Verification items for the finished model (mm, model axes). Face numbers are marked on the shaded views. A direction names the side the tool comes from. Give positions to 0.01 mm unless a question says otherwise; leave off trailing zeros. Write each loop counter-clockwise with the first axis right and the second up, starting at its lowest first coordinate (ties: lowest second). Pieces come first, ordered by that corner, then holes. Notation, with made-up numbers: (-32, 58) - (22, 58) arc R9 ccw to (22, 62) - close; hole circle Ø4 at (-4, 70). An arc over 180 degrees is marked (long way). Answer as a JSON object with one key per item and string values. Group by question number.
Item 1: Sectioned sample at D-D, the plane y = 26. Record the boundary of the cut face in (x, z), and give its area (3 significant figures).
Item 2: Draft check along X on the marked faces 1, 2, 3 and 4. Enter one of: +X half, -X half, draft (parallel to the pull), parting line (faces both ways), or undercut.
Item 3: Scan lines: line 1 along Z through (x, y) = (81.5, -1.5); line 2 along X through (y, z) = (13.5, -5.5); line 3 along Y through (x, z) = (38.5, -37.5). Record each from-to range of solid material in increasing order. Write a range as [from, to].
Item 4: Tool access check on the marked faces 5, 6 and 7. Record the directions out of +Z, -Z, +X, -X, +Y, -Y that give a thin tool (end or side, any length) a straight path to the whole face; none if there is none.
Item 5: Sectioned sample at A-A, the plane y = 56.5. Record the boundary of the cut face in (x, z), and give its area (3 significant figures).
Item 6: Sectioned sample at B-B, the plane x = 50. Record the boundary of the cut face in (y, z).
Item 7: Sectioned sample at C-C, the plane z = -7. Record the boundary of the cut face in (x, y).
Item 8: Go/stop test with flat-tipped pins: pin 1 (8 mm diameter, centred on x = -108, z = -33, fed in from +Y); pin 2 (3 mm diameter, centred on x = -90.5, y = 8, fed in from -Z); pin 3 (10 mm diameter, centred on x = -123.5, y = -10.5, fed in from -Z); pin 4 (6 mm diameter, centred on x = 107.73, z = 16.4, fed in from -Y). Record where each tip stops, or that it passes through.
```python
from build123d import *

# Parameters (mm, degrees)
BOSS_EXTRUDE1_DEPTH = 10
CUT_EXTRUDE1_DEPTH  = 9.5
SKETCH3_R           = 0.15
SKETCH3_R_2         = 0.5
CUT_EXTRUDE2_DEPTH  = 20.798989873
SKETCH4_R           = 0.1
SKETCH4_W           = 8.7
SKETCH4_H           = 5.3
CUT_EXTRUDE3_DEPTH  = 20.798989873
CUT_EXTRUDE5_REACH  = 24.361
SKETCH5_W           = 20
SKETCH5_H           = 9
BOSS_EXTRUDE5_START = 9.5
SKETCH6_W           = 3.5
SKETCH6_H           = 1
BOSS_EXTRUDE5_DEPTH = 9.5
SCALE2_SCALE        = 10
SKETCH9_R           = 1.5
CUT_EXTRUDE6_DEPTH  = 10


with BuildPart() as part:
    # Sketch1 → Boss-Extrude1 (new body)
    with BuildSketch(Plane(origin=(0, 0, 0), x_dir=(1, 0, 0), z_dir=(0, 1, 0))):
        with BuildLine():
            Line((-10, 6), (10, 6))
            ThreePointArc((10, 6), (16, 0), (10, -6))
            Line((10, -6), (-10, -6))
            ThreePointArc((-10, -6), (-16, 0), (-10, 6))
        make_face()
    extrude(amount=BOSS_EXTRUDE1_DEPTH)

    # Sketch2 → Cut-Extrude1 (cut)
    with BuildSketch(Plane(origin=(0, 10, 0), x_dir=(1, 0, 0), z_dir=(0, 1, 0))):
        with BuildLine():
            Line((-10, 5.5), (10, 5.5))
            ThreePointArc((10, 5.5), (15.5, 0), (10, -5.5))
            Line((10, -5.5), (-10, -5.5))
            ThreePointArc((-10, -5.5), (-15.5, 0), (-10, 5.5))
        make_face()
    extrude(amount=-CUT_EXTRUDE1_DEPTH, mode=Mode.SUBTRACT)

    # Sketch3 → Cut-Extrude2 (cut, through all)
    with BuildSketch(Plane.XZ):
        with Locations(Location((-13, 3, 0), (0, 0, 270))):
            Circle(SKETCH3_R)
        with Locations(Location((-7, 3, 0), (0, 0, 270))):
            Circle(SKETCH3_R)
        with Locations(Location((-13, -3, 0), (0, 0, 270))):
            Circle(SKETCH3_R)
        with Locations(Location((-7, -3, 0), (0, 0, 270))):
            Circle(SKETCH3_R)
        with Locations(Location((-12.5, 0, 0), (0, 0, 270))):
            Circle(SKETCH3_R_2)
        with Locations(Location((-12.022542486, 1.469463131, 0), (0, 0, 270))):
            Circle(SKETCH3_R_2)
        with Locations(Location((-10.772542486, 2.377641291, 0), (0, 0, 270))):
            Circle(SKETCH3_R_2)
        with Locations(Location((-9.227457514, 2.377641291, 0), (0, 0, 270))):
            Circle(SKETCH3_R_2)
        with Locations(Location((-7.977457514, 1.469463131, 0), (0, 0, 270))):
            Circle(SKETCH3_R_2)
        with Locations(Location((-7.5, 0, 0), (0, 0, 270))):
            Circle(SKETCH3_R_2)
        with Locations(Location((-7.977457514, -1.469463131, 0), (0, 0, 270))):
            Circle(SKETCH3_R_2)
        with Locations(Location((-9.227457514, -2.377641291, 0), (0, 0, 270))):
            Circle(SKETCH3_R_2)
        with Locations(Location((-10.772542486, -2.377641291, 0), (0, 0, 270))):
            Circle(SKETCH3_R_2)
        with Locations(Location((-12.022542486, -1.469463131, 0), (0, 0, 270))):
            Circle(SKETCH3_R_2)
        with Locations(Location((12.022542486, -1.469463131, 0), (0, 0, 90))):
            Circle(SKETCH3_R_2)
        with Locations(Location((10.772542486, -2.377641291, 0), (0, 0, 90))):
            Circle(SKETCH3_R_2)
        with Locations(Location((9.227457514, -2.377641291, 0), (0, 0, 90))):
            Circle(SKETCH3_R_2)
        with Locations(Location((7.977457514, -1.469463131, 0), (0, 0, 90))):
            Circle(SKETCH3_R_2)
        with Locations(Location((7.5, 0, 0), (0, 0, 90))):
            Circle(SKETCH3_R_2)
        with Locations(Location((7.977457514, 1.469463131, 0), (0, 0, 90))):
            Circle(SKETCH3_R_2)
        with Locations(Location((9.227457514, 2.377641291, 0), (0, 0, 90))):
            Circle(SKETCH3_R_2)
        with Locations(Location((10.772542486, 2.377641291, 0), (0, 0, 90))):
            Circle(SKETCH3_R_2)
        with Locations(Location((12.022542486, 1.469463131, 0), (0, 0, 90))):
            Circle(SKETCH3_R_2)
        with Locations(Location((12.5, 0, 0), (0, 0, 90))):
            Circle(SKETCH3_R_2)
        with Locations(Location((7, -3, 0), (0, 0, 90))):
            Circle(SKETCH3_R)
        with Locations(Location((13, -3, 0), (0, 0, 90))):
            Circle(SKETCH3_R)
        with Locations(Location((7, 3, 0), (0, 0, 90))):
            Circle(SKETCH3_R)
        with Locations(Location((13, 3, 0), (0, 0, 90))):
            Circle(SKETCH3_R)
    extrude(amount=-CUT_EXTRUDE2_DEPTH, mode=Mode.SUBTRACT)

    # Sketch4 → Cut-Extrude3 (cut, through all)
    with BuildSketch(Plane.XZ):
        with Locations(Location((-4.572, 2.794, 0), (0, 0, 270))):
            Circle(SKETCH4_R)
        with Locations(Location((4.572, 2.794, 0), (0, 0, 270))):
            Circle(SKETCH4_R)
        with Locations(Location((-4.572, -2.794, 0), (0, 0, 270))):
            Circle(SKETCH4_R)
        with Locations(Location((4.572, -2.794, 0), (0, 0, 270))):
            Circle(SKETCH4_R)
        Rectangle(SKETCH4_W, SKETCH4_H)
    extrude(amount=-CUT_EXTRUDE3_DEPTH, mode=Mode.SUBTRACT)

    # Cut-Extrude5: up to this face of the body (flat: up to its plane)
    cut_extrude5_end = Plane(part.part.faces().sort_by_distance((0, 5.25, -5.5))[0])
    # Sketch5 → Cut-Extrude5 (cut, up to the picked face)
    with BuildSketch(Plane(origin=(0, 0, -6), x_dir=(-1, 0, 0), z_dir=(0, 0, -1)), mode=Mode.PRIVATE) as cut_extrude5_sk1:
        with Locations((0, 5.5)):
            Rectangle(SKETCH5_W, SKETCH5_H)
    cut_extrude5_tool1 = split(extrude(cut_extrude5_sk1.sketch, amount=-CUT_EXTRUDE5_REACH, mode=Mode.PRIVATE), bisect_by=cut_extrude5_end, keep=Keep.BOTH, mode=Mode.PRIVATE)
    add(cut_extrude5_tool1.solids().sort_by(Axis((0, 5.5, -6), (0, 0, 1)))[0], mode=Mode.SUBTRACT)

    # Sketch6 → Boss-Extrude5 (add)
    with BuildSketch(Plane(origin=(0, 0.5, 0), x_dir=(1, 0, 0), z_dir=(0, 1, 0)).offset(BOSS_EXTRUDE5_START)):
        with Locations((8.25, -5)):
            Rectangle(SKETCH6_W, SKETCH6_H)
        with Locations((8.25, 5)):
            Rectangle(SKETCH6_W, SKETCH6_H)
        with BuildLine():
            ThreePointArc((13.16227766, 4.5), (11.658312395, 5.244044241), (10, 5.5))
            Line((10, 5.5), (10, 4.5))
            Line((10, 4.5), (13.16227766, 4.5))
        make_face()
        with BuildLine():
            ThreePointArc((10, -5.5), (11.658312395, -5.244044241), (13.16227766, -4.5))
            Line((13.16227766, -4.5), (10, -4.5))
            Line((10, -4.5), (10, -5.5))
        make_face()
        with Locations((-8.25, -5)):
            Rectangle(SKETCH6_W, SKETCH6_H)
        with Locations((-8.25, 5)):
            Rectangle(SKETCH6_W, SKETCH6_H)
        with BuildLine():
            Line((-10, 4.5), (-10, 5.5))
            ThreePointArc((-10, 5.5), (-11.658312395, 5.244044241), (-13.16227766, 4.5))
            Line((-13.16227766, 4.5), (-10, 4.5))
        make_face()
        with BuildLine():
            Line((-10, -4.5), (-13.16227766, -4.5))
            ThreePointArc((-13.16227766, -4.5), (-11.658312395, -5.244044241), (-10, -5.5))
            Line((-10, -5.5), (-10, -4.5))
        make_face()
    extrude(amount=-BOSS_EXTRUDE5_DEPTH)


with BuildPart() as part_1:
    # Scale2: scaled about (0, 4.064159542, 0.819354557)
    add(part.part.scale(SCALE2_SCALE).moved(Location((0, -36.577435878, -7.374191013))))

    # Sketch9 → Cut-Extrude6 (cut)
    with BuildSketch(Plane(origin=(0, 63.422564119, 0), x_dir=(1, 0, 0), z_dir=(0, 1, 0))):
        with Locations(Location((-110, 57.374191011, 0), (0, 0, 270))):
            Circle(SKETCH9_R)
        with Locations(Location((-110, -42.625808989, 0), (0, 0, 270))):
            Circle(SKETCH9_R)
        with Locations(Location((110, -42.625808989, 0), (0, 0, 270))):
            Circle(SKETCH9_R)
        with Locations(Location((110, 57.374191011, 0), (0, 0, 270))):
            Circle(SKETCH9_R)
    extrude(amount=-CUT_EXTRUDE6_DEPTH, mode=Mode.SUBTRACT)


solid = part_1.part
```
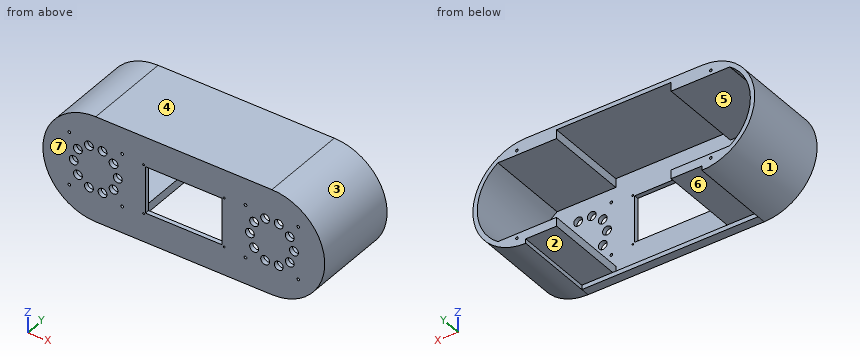
Geometry check:
{
 "1": {"outline": "(-131.62, -52.37) arc R55 cw to (-131.62, 37.63) - (-65, 37.63) - (-65, 47.63) - (65, 47.63) - (65, 37.63) - (131.62, 37.63) arc R55 cw to (131.62, -52.37) - (65, -52.37) - (65, -62.37) - (100, -62.37) - (100, -67.37) arc R60 ccw to (100, 52.63) - (-100, 52.63) arc R60 ccw to (-100, -67.37) - (-100, -62.37) - (-65, -62.37) - (-65, -52.37) - close", "area": "5,070 mm^2"},
 "2": {"face 1": "-X half", "face 2": "undercut", "face 3": "+X half", "face 4": "draft"},
 "3": {"line 1": "[-62.37, -52.37], [37.63, 52.63]", "line 2": "[-159.97, -154.97], [154.97, 159.97]", "line 3": "[-36.58, -31.58]"},
 "4": {"face 5": "+Y", "face 6": "-Z, +Y", "face 7": "+Z, -Z, +X, -X, -Y"},
 "5": {"outline": "(-131.62, -52.37) arc R55 cw to (-131.62, 37.63) - (-65, 37.63) - (-65, 47.63) - (65, 47.63) - (65, 37.63) - (131.62, 37.63) arc R55 cw to (131.62, -52.37) - (65, -52.37) - (65, -62.37) - (100, -62.37) - (100, -67.37) arc R60 ccw to (100, 52.63) - (-100, 52.63) arc R60 ccw to (-100, -67.37) - (-100, -62.37) - (-65, -62.37) - (-65, -52.37) - close; hole circle Ø3 at (-110, -57.37); hole circle Ø3 at (-110, 42.63); hole circle Ø3 at (110, -57.37); hole circle Ø3 at (110, 42.63)", "area": "5,040 mm^2"},
 "6": {"outline": "(-36.58, -67.37) - (-26.58, -67.37) - (-26.58, -62.37) - (-31.58, -62.37) - (-31.58, 47.63) - (63.42, 47.63) - (63.42, 52.63) - (-36.58, 52.63) - close"},
 "7": {"outline": "(-160, -36.58) - (-129.99, -36.58) - (-129.99, -31.58) - (-155, -31.58) - (-155, 63.42) - (-160, 63.42) - close; (-120.01, -36.58) - (-79.99, -36.58) - (-79.99, -31.58) - (-120.01, -31.58) - close; (-70.01, -36.58) - (-43.5, -36.58) - (-43.5, -31.58) - (-70.01, -31.58) - close; (43.5, -36.58) - (70.01, -36.58) - (70.01, -31.58) - (43.5, -31.58) - close; (79.99, -36.58) - (120.01, -36.58) - (120.01, -31.58) - (79.99, -31.58) - close; (129.99, -36.58) - (160, -36.58) - (160, 63.42) - (155, 63.42) - (155, -31.58) - (129.99, -31.58) - close"},
 "8": {"pin 1": "y = -31.58", "pin 2": "z = -62.37", "pin 3": "z = -64.45", "pin 4": "through"}
}
